```python
from build123d import *

# Parameters (mm, degrees)
CROQUIS1_R              = 35
SALIENTE_EXTRUIR1_DEPTH = 90
SALIENTE_EXTRUIR2_DEPTH = 30
CROQUIS3_W              = 40
CROQUIS3_H              = 20
CORTAR_EXTRUIR1_DEPTH   = 28


with BuildPart() as part:
    # Croquis1 → Saliente-Extruir1 (new body)
    with BuildSketch(Plane(origin=(0, 0, 0), x_dir=(1, 0, 0), z_dir=(0, 1, 0))):
        with Locations(Location((0, 0, 0), (0, 0, 90))):
            Circle(CROQUIS1_R)
    extrude(amount=SALIENTE_EXTRUIR1_DEPTH)

    # Croquis2 → Saliente-Extruir2 (add)
    with BuildSketch(Plane.XZ):
        with BuildLine():
            Line((50, 60), (50, -60))
            Line((50, -60), (32.42606327, -60))
            ThreePointArc((32.42606327, -60), (30.068391754, -59.718095751), (27.843647762, -58.888277005))
            Line((27.843647762, -58.888277005), (-18.138307464, -35.181947356))
            ThreePointArc((-18.138307464, -35.181947356), (-39.582415507, 0), (-18.138307464, 35.181947356))
            Line((-18.138307464, 35.181947356), (27.843647762, 58.888277005))
            ThreePointArc((27.843647762, 58.888277005), (30.068391754, 59.718095751), (32.42606327, 60))
            Line((32.42606327, 60), (50, 60))
        make_face()
    extrude(amount=-SALIENTE_EXTRUIR2_DEPTH)

    # Croquis3 → Cortar-Extruir1 (cut)
    with BuildSketch(Plane(origin=(50, 0, 0), x_dir=(0, 0, -1), z_dir=(1, 0, 0))):
        with Locations((-35, 15)):
            Rectangle(CROQUIS3_W, CROQUIS3_H)
        with Locations((35, 15)):
            Rectangle(CROQUIS3_W, CROQUIS3_H)
    extrude(amount=-CORTAR_EXTRUIR1_DEPTH, mode=Mode.SUBTRACT)


solid = part.part
```
Model file for the job. Use its own axes, mm. A direction names the side the tool comes from. Coordinates: 2 decimals unless noted, no trailing zeros. Write each loop counter-clockwise with the first axis right and the second up, starting at its lowest first coordinate (ties: lowest second). Pieces come first, ordered by that corner, then holes. Notation, with made-up numbers: (62.5, 25) - (92.5, 25) arc R18 ccw to (92.5, 55) - close; hole circle Ø6 at (85, 58.25). An arc over 180 degrees is marked (long way). One line per item, written item: value. Start each with the question number.
1. Slice it at C-C (x = 0). Write the cut outline in (y, z), plus the area to 3 significant figures.
2. Slice it at A-A (y = 17). Write the cut outline in (x, z), plus the area to 3 significant figures.
3. Flat gauge pins, fed straight in: pin 1 (8.5 mm diameter, centred on x = 30, z = 39, fed in from +Y); pin 2 (12 mm diameter, centred on x = 10.5, y = 55.5, fed in from -Z); pin 3 (4 mm diameter, centred on x = -16.5, y = 57, fed in from +Z). Where does each tip first touch, or does it go through?
4. Mould opens along Z. For faces 4 (the cylindrical face through (-39.578, 14.79, -0.607)), 5 (the flat face through (36, 25, -35)), 6 (the flat face through (0, 90, 0)) say: released by +Z, released by -Z, zero draft, split by the parting line, or undercut.
5. Slice it at B-B (z = 0). Write the cut outline in (x, y).
6. Slice it at D-D (z = -26). Write the cut outline in (x, y), plus the area to 3 significant figures.
7. Probe line 1 (Z direction, x = 46.5, y = 13.5); line 2 (Y direction, x = 39, z = 23); line 3 (X direction, y = 51, z = -1). List the from-to ranges inside material, lowest first. Write a range as from..to.
8. Tool access for faces 1 (the cylindrical face through (21, 60, 28)), 2 (the flat face through (36, 15, 15)), 3 (the flat face through (5.17, 14.79, -47.2)): list every direction of +Z, -Z, +X, -X, +Y, -Y with a clear straight run to the whole face (end or side of a thin tool).
Answers below:
1. outline: (0, -44.53) - (30, -44.53) - (30, -35) - (90, -35) - (90, 35) - (30, 35) - (30, 44.53) - (0, 44.53) - close
1. area: 6,870 mm^2
2. outline: (-18.14, -35.18) - (27.84, -58.89) arc R10 ccw to (32.43, -60) - (50, -60) - (50, -55) - (22, -55) - (22, -15) - (50, -15) - (50, 15) - (22, 15) - (22, 55) - (50, 55) - (50, 60) - (32.43, 60) arc R10 ccw to (27.84, 58.89) - (-18.14, 35.18) arc R39.58 ccw to start
2. area: 5,820 mm^2
3. pin 1: stops at y = 30
3. pin 2: stops at z = -34.71
3. pin 3: stops at z = 31.86
4. face 4: split by the parting line
4. face 5: undercut
4. face 6: zero draft
5. outline: (-39.58, 0) - (50, 0) - (50, 30) - (35, 30) - (35, 90) - (-35, 90) - (-35, 30) - (-39.58, 30) - close
6. outline: (-29.85, 0) - (50, 0) - (50, 5) - (22, 5) - (22, 25) - (50, 25) - (50, 30) - (23.43, 30) - (23.43, 90) - (-23.43, 90) - (-23.43, 30) - (-29.85, 30) - close
6. area: 4,650 mm^2
7. line 1: z = -60..-55, -15..15, 55..60
7. line 2: y = 0..5, 25..30
7. line 3: x = -34.99..34.99
8. face 1: +Y
8. face 2: +X
8. face 3: -Z, -X, +Y, -Y
